Geometry check sheet. Reference: the model listing, model coordinates, mm. A direction names the side the tool comes from. Give positions to 0.01 mm unless a question says otherwise; leave off trailing zeros. Loops run counter-clockwise (first coordinate to the right, second up) from the corner with the lowest first, then second, coordinate; pieces in that order, holes last. Notation, with made-up numbers: (-12.75, 42.25) -> (25.25, 42.25) arc R8 cw to (25.25, 53.25) -> close; hole circle Ø1 at (57.5, 15.5). An arc over 180 degrees is marked (long way). Write item = value, one per line.
```python
from build123d import *

# Parameters (mm, degrees)
F0_W     = 152.4
F0_H     = 12.7
F1_DEPTH = 165.1
F2_SIZE2 = 101.6
F2_SIZE  = 76.2
F4_DEPTH = 19.812
F6_DEPTH = 25.4


with BuildPart() as f1:
    # F0 (on Top) → F1 (new body)
    with BuildSketch(Plane.XY):
        Rectangle(F0_W, F0_H)
    extrude(amount=-F1_DEPTH)

    # F2
    f2_edges = [f1.edges().sort_by_distance(p)[0] for p in [
        (76.2, 0, 0),
    ]]
    chamfer(f2_edges, length=F2_SIZE, length2=F2_SIZE2)

    # F3 (on face) → F4 (join)
    with BuildSketch(Plane.XZ.offset(6.35)):
        Polygon((-2.6924, -165.1), (76.2, -165.1), (76.2, -120.65), (76.2, -76.2), (-2.6924, -76.2), align=None)
    extrude(amount=F4_DEPTH)

    # F5 (on face) → F6 (cut)
    with BuildSketch(Plane(origin=(0, 6.35, 0), x_dir=(-1, 0, 0), z_dir=(0, 1, 0))):
        Polygon((-8.466667, -25.4), (-76.2, -76.2), (-8.466667, -76.2), align=None)
    extrude(amount=-F6_DEPTH, mode=Mode.SUBTRACT)


solid = f1.part
```
Item 1: Tool access check on faces 1 (the flat face through (-51, 0, 0)), 2 (the flat face through (-2.692, -16, -120)), 3 (the flat face through (8.467, 0, -51)). Record the directions out of +Z, -Z, +X, -X, +Y, -Y that give a thin tool (end or side, any length) a straight path to the whole face; none if there is none.
Answer:
face_1 = +Z, +X, -X, +Y, -Y
face_2 = +Z, -Z, -X, -Y
face_3 = +Z, +X, +Y, -Y
Item 2: Section check B-B, the plane z = -107. Record the cut outline in (x, y), plus the area to 3 significant figures.
Answer:
outline = (-76.2, -6.35) -> (-2.69, -6.35) -> (-2.69, -26.16) -> (76.2, -26.16) -> (76.2, 6.35) -> (-76.2, 6.35) -> close
area = 3,500 mm^2
Item 3: Section check A-A, the plane y = -4. Record the cut outline in (x, z), plus the area to 3 significant figures.
Answer:
outline = (-76.2, -165.1) -> (76.2, -165.1) -> (76.2, -76.2) -> (8.47, -76.2) -> (8.47, -25.4) -> (-25.4, 0) -> (-76.2, 0) -> close
area = 19,600 mm^2
Item 4: Section check D-D, the plane x = 2.5. Record the cut outline in (y, z) (3 decimals).
Answer:
outline = (-26.162, -165.1) -> (6.35, -165.1) -> (6.35, -20.925) -> (-6.35, -20.925) -> (-6.35, -76.2) -> (-26.162, -76.2) -> close
Item 5: Gauge pin test, flat ends, axial feed: pin 1 (4 mm diameter, centred on y = -2, z = -39.5, fed in from +X); pin 2 (1.5 mm diameter, centred on x = -40.5, z = -101, fed in from -Y); pin 3 (10 mm diameter, centred on x = 22.5, y = -15, fed in from +Z). Record the tip position at first contact, or that the pin passes through.
Answer:
pin_1 = 8.47
pin_2 = -6.35
pin_3 = -76.2
Item 6: Thickness scan on L1, parallel to Z at x = 70.5, y = -9.5; L2, parallel to X at y = -2, z = -59.5; L3, parallel to Y at x = -40, z = -105. Record the ranges inside material, lowest first. Write a range as [from, to].
Answer:
L1 = [-165.1, -76.2]
L2 = [-76.2, 8.47]
L3 = [-6.35, 6.35]
Item 7: Section check C-C, the plane x = 29. Record the cut outline in (y, z), plus the area to 3 significant figures.
Answer:
outline = (-26.16, -165.1) -> (6.35, -165.1) -> (6.35, -76.2) -> (-26.16, -76.2) -> close
area = 2,890 mm^2
